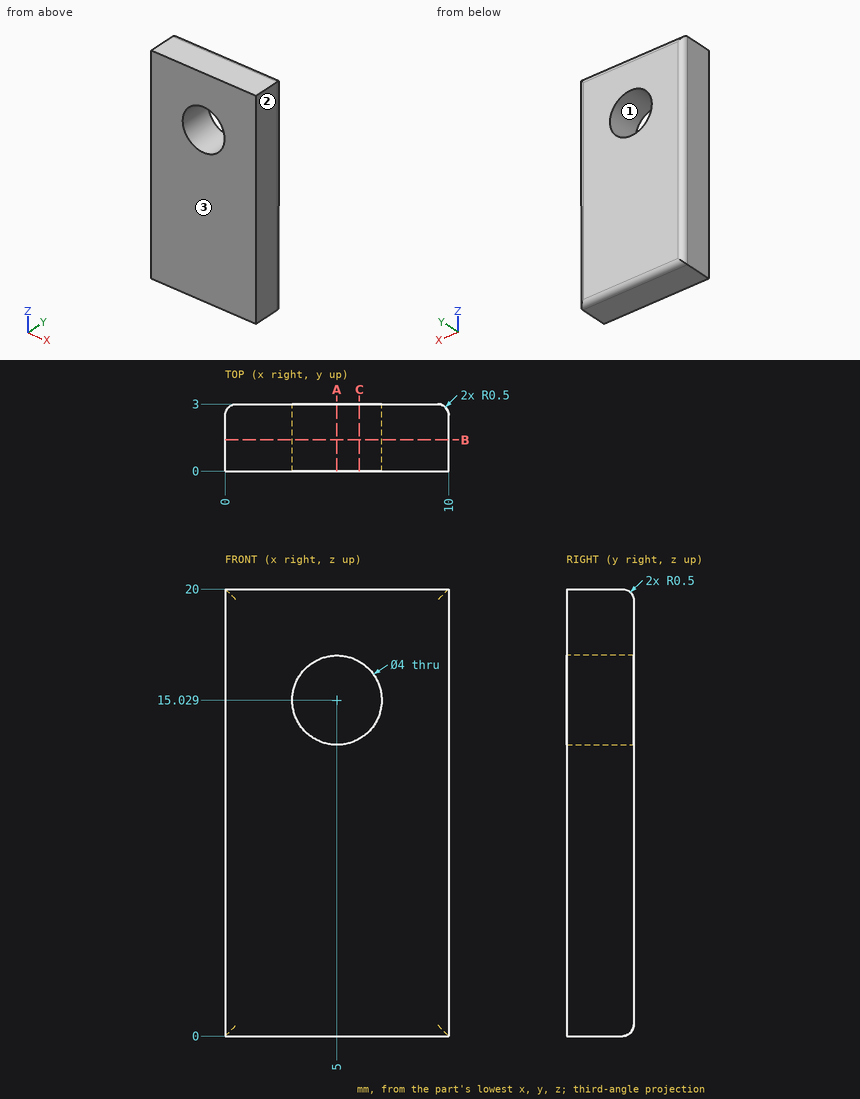
Part print with two shaded views. Sizes in mm from the minimum x, y, z corner. Give positions to 0.01 mm unless a question says otherwise; leave off trailing zeros. Loops run counter-clockwise (first coordinate to the right, second up) from the corner with the lowest first, then second, coordinate; pieces in that order, holes last. Notation, with made-up numbers: (73.5, -32.75) - (131.5, -32.75) arc R14 ccw to (131.5, -23.75) - close; hole circle Ø3 at (34, 17.5). An arc over 180 degrees is marked (long way). Put each result on its own line as item: value.
Q1. Slice it at A-A (x = 5). Give the cut face in (y, z).
Filled in:
outline: (0, 0) - (2.5, 0) arc R0.5 ccw to (3, 0.5) - (3, 13.03) - (0, 13.03) - close; (0, 17.03) - (3, 17.03) - (3, 19.5) arc R0.5 ccw to (2.5, 20) - (0, 20) - close
Q2. Slice it at B-B (y = 1.4). Give the cut face in (x, z).
Filled in:
outline: (0, 0) - (10, 0) - (10, 20) - (0, 20) - close; hole circle Ø4 at (5, 15.03)
Q3. Probe line 1 along Z through (x, y) = (3.5, 1.2); line 2 along X through (y, z) = (2.5, 16); line 3 along X through (y, z) = (2.3, 15.75). List the from-to ranges inside material, lowest first.
Filled in:
line 1: z = 0 to 13.71, 16.35 to 20
line 2: x = 0 to 3.25, 6.75 to 10
line 3: x = 0 to 3.13, 6.87 to 10
Q4. Mould opens along X. For the marked faces 1, 2 and 3 say: pulls with the +X half, pulls with the -X half, needs draft (parallel to the pull), parting line crosses it, or undercut.
Filled in:
face 1: undercut
face 2: pulls with the +X half
face 3: needs draft
Q5. Slice it at C-C (x = 6). Give the cut face in (y, z), plus the area to 3 significant figures.
Filled in:
outline: (0, 0) - (2.5, 0) arc R0.5 ccw to (3, 0.5) - (3, 13.3) - (0, 13.3) - close; (0, 16.76) - (3, 16.76) - (3, 19.5) arc R0.5 ccw to (2.5, 20) - (0, 20) - close
area: 49.5 mm²
